Can you work these out from the model? Positions are in its coordinate system, mm. Face numbers are marked on the shaded views. A direction names the side the tool comes from. Give positions to 0.01 mm unless a question says otherwise; leave off trailing zeros. Loops run counter-clockwise (first coordinate to the right, second up) from the corner with the lowest first, then second, coordinate; pieces in that order, holes last. Notation, with made-up numbers: (84, -6) - (122, -6) arc R24 cw to (122, 15) - close; hole circle Ø2 at (-39, -20). An arc over 180 degrees is marked (long way). Answer in a Markdown table with one row per item.
from build123d import *

# Parameters (mm, degrees)
F1_DEPTH = 101.6
F3_DEPTH = 50.8
F4_W     = 50.8
F4_H     = 50.8
F5_DEPTH = 152.401


with BuildPart() as f1:
    # F0 (on Top) → F1 (new body)
    with BuildSketch(Plane.XY):
        Polygon((101.6, 0), (0, 0), (0, -101.6), align=None)
    extrude(amount=F1_DEPTH)

    # F2 (on face) → F3 (join)
    with BuildSketch(Plane.XY.offset(101.6)):
        Polygon((101.6, 0), (0, 0), (0, -101.6), align=None)
        Polygon((101.6, -101.6), (101.6, 0), (0, -101.6), align=None)
    extrude(amount=F3_DEPTH)

    # F4 (on face) → F5 (cut, through all)
    with BuildSketch(Plane.XY.offset(152.4)):
        with Locations((76.2, -76.2)):
            Rectangle(F4_W, F4_H)
    extrude(amount=-F5_DEPTH, mode=Mode.SUBTRACT)


solid = f1.part
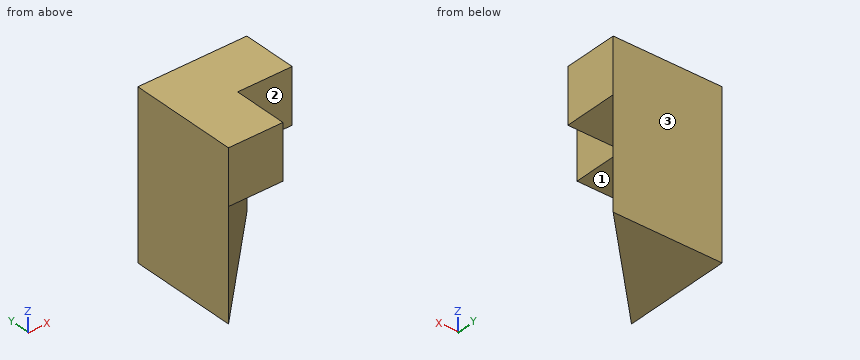
Q1. If I drill on line 1 (Z direction, x = 37, y = -82); line 2 (X direction, y = -91, z = 124.5); line 3 (Y direction, x = 91, z = 108), over which ranges is the centre line in solid material (lowest first)? Write a range as [from, to].
Checked values:
| item | result |
|---|---|
| line 1 | z = [101.6, 152.4] |
| line 2 | x = [0, 50.8] |
| line 3 | y = [-50.8, 0] |
Q2. On a 3-axis mill with a long thin cutter (end or side, diameter ignored), from which of +Z, -Z, +X, -X, +Y, -Y can I reach the whole of each face in a straight line? I mean the marked faces 1, 2 and 3. Say none if no direction works.
Checked values:
| item | result |
|---|---|
| face 1 | -Z, +X, -Y |
| face 2 | +Z, -Z, +X, -Y |
| face 3 | +Z, -Z, +X, -X, +Y |
Q3. For pin 1 (5 mm diameter, centred on y = -51, z = 36.5, fed in from +X); pin 2 (4 mm diameter, centred on x = 72.5, z = 116.5, fed in from -Y); pin 3 (3 mm diameter, centred on x = 77, y = -41, fed in from -Z), each with a flat end and sliding along its axis, tell me the tip position at first contact or that it passes through.
Checked values:
| item | result |
|---|---|
| pin 1 | stops at x = 53.1 |
| pin 2 | stops at y = -50.8 |
| pin 3 | stops at z = 101.6 |
Q4. Imagine slicing it at C-C, the plane z = 64.5. Write out the boundary of the cut face in (x, y).
Checked values:
| item | result |
|---|---|
| outline | (0, -101.6) - (101.6, 0) - (0, 0) - close |
Q5. Imagine slicing it at B-B, the plane y = -44.5. Write out the boundary of the cut face in (x, z).
Checked values:
| item | result |
|---|---|
| outline | (0, 0) - (57.1, 0) - (57.1, 101.6) - (101.6, 101.6) - (101.6, 152.4) - (0, 152.4) - close |
Q6. Imagine slicing it at A-A, the plane x = 40. Write out the boundary of the cut face in (y, z), and give its area (3 significant figures).
Checked values:
| item | result |
|---|---|
| outline | (-101.6, 101.6) - (-61.6, 101.6) - (-61.6, 0) - (0, 0) - (0, 152.4) - (-101.6, 152.4) - close |
| area | 11,400 mm² |
